Here's how the part is built. I have some questions about the finished solid (model axes, mm). Give positions to 0.01 mm unless a question says otherwise; leave off trailing zeros. Write each loop counter-clockwise with the first axis right and the second up, starting at its lowest first coordinate (ties: lowest second). Pieces come first, ordered by that corner, then holes. Notation, with made-up numbers: (-16.75, 33.25) -> (14.25, 33.25) arc R14 cw to (14.25, 46.25) -> close; hole circle Ø9 at (38, 68.5). An arc over 180 degrees is marked (long way). Return JSON: item names as keys, results as strings.
from build123d import *

# Parameters (mm, degrees)
CROQUIS1_R              = 12.5
CROQUIS1_R_2            = 5.125
SALIENTE_EXTRUIR1_DEPTH = 1


with BuildPart() as part:
    # Croquis1 → Saliente-Extruir1 (new body)
    with BuildSketch(Plane(origin=(0, 0, 0), x_dir=(1, 0, 0), z_dir=(0, 1, 0))):
        with Locations(Location((0, 0, 0), (0, 0, 270))):
            Circle(CROQUIS1_R)
        with Locations(Location((0, 0, 0), (0, 0, 270))):
            Circle(CROQUIS1_R_2, mode=Mode.SUBTRACT)
        with BuildLine():
            ThreePointArc((5.375, 9.309773091), (0, 10.75), (-5.375, 9.309773091))
            ThreePointArc((-5.375, 9.309773091), (-6.015544457, 6.919228634), (-3.625, 6.278684177))
            ThreePointArc((-3.625, 6.278684177), (0, 7.25), (3.625, 6.278684177))
            ThreePointArc((3.625, 6.278684177), (6.015544457, 6.919228634), (5.375, 9.309773091))
        make_face(mode=Mode.SUBTRACT)
        with BuildLine():
            ThreePointArc((5.375, -9.309773091), (9.309773091, -5.375), (10.75, 0))
            ThreePointArc((10.75, 0), (9, 1.75), (7.25, 0))
            ThreePointArc((7.25, 0), (6.278684177, -3.625), (3.625, -6.278684177))
            ThreePointArc((3.625, -6.278684177), (2.984455543, -8.669228634), (5.375, -9.309773091))
        make_face(mode=Mode.SUBTRACT)
        with BuildLine():
            ThreePointArc((-10.75, 0), (-9.309773091, -5.375), (-5.375, -9.309773091))
            ThreePointArc((-5.375, -9.309773091), (-2.984455543, -8.669228634), (-3.625, -6.278684177))
            ThreePointArc((-3.625, -6.278684177), (-6.278684177, -3.625), (-7.25, 0))
            ThreePointArc((-7.25, 0), (-9, 1.75), (-10.75, 0))
        make_face(mode=Mode.SUBTRACT)
    extrude(amount=SALIENTE_EXTRUIR1_DEPTH)


solid = part.part
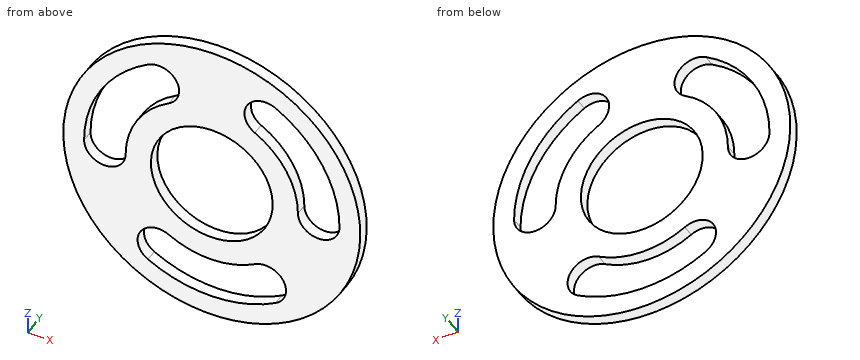
1. If I drill on line 1 (Z direction, x = -6, y = 0.75); line 2 (Z direction, x = -4.5, y = 0.65); line 3 (X direction, y = 0.95, z = 4.5), over which ranges is the centre line in solid material (lowest first)? Write a range as [from, to].
Taken from the geometry:
{"line 1": "z = [-10.97, -8.7], [-6.89, 4.07], [8.92, 10.97]", "line 2": "z = [-11.66, -9.76], [-6.04, -2.45], [2.45, 5.68], [9.54, 11.66]", "line 3": "x = [-11.66, -9.76], [-5.68, -2.45], [2.45, 5.68], [9.76, 11.66]"}
2. Suppose I cut it at D-D, the plane x = -8.5. List the corners of the cut face in (y, z) for me.
Taken from the geometry:
{"outline": "(0, -9.17) -> (1, -9.17) -> (1, -1.68) -> (0, -1.68) -> close; (0, 6.58) -> (1, 6.58) -> (1, 9.17) -> (0, 9.17) -> close"}
3. Suppose I cut it at A-A, the plane y = 0.4. List the corners of the cut face in (x, z) for me (3 decimals).
Taken from the geometry:
{"outline": "circle Ø25 at (0, 0); hole (-10.75, 0) arc R1.75 ccw to (-7.25, 0) arc R7.25 cw to (-3.625, 6.279) arc R1.75 ccw to (-5.375, 9.31) arc R10.75 ccw to start; hole (-5.375, -9.31) arc R10.75 ccw to (5.375, -9.31) arc R1.75 ccw to (3.625, -6.279) arc R7.25 cw to (-3.625, -6.279) arc R1.75 ccw to start; hole circle Ø10.25 at (0, 0); hole (3.625, 6.279) arc R7.25 cw to (7.25, 0) arc R1.75 ccw to (10.75, 0) arc R10.75 ccw to (5.375, 9.31) arc R1.75 ccw to start"}
4. Suppose I cut it at C-C, the plane x = 4.25. List the corners of the cut face in (y, z) for me, and give its area (3 significant figures).
Taken from the geometry:
{"outline": "(0, -11.76) -> (1, -11.76) -> (1, -9.87) -> (0, -9.87) -> close; (0, -6.06) -> (1, -6.06) -> (1, -2.86) -> (0, -2.86) -> close; (0, 2.86) -> (1, 2.86) -> (1, 5.87) -> (0, 5.87) -> close; (0, 9.53) -> (1, 9.53) -> (1, 11.76) -> (0, 11.76) -> close", "area": "10.3 mm²"}
5. Suppose I cut it at B-B, the plane x = 0. List the corners of the cut face in (y, z) for me (3 decimals).
Taken from the geometry:
{"outline": "(0, -12.5) -> (1, -12.5) -> (1, -10.75) -> (0, -10.75) -> close; (0, -7.25) -> (1, -7.25) -> (1, -5.125) -> (0, -5.125) -> close; (0, 5.125) -> (1, 5.125) -> (1, 12.5) -> (0, 12.5) -> close"}
